Source: three-view drawing plus pictorial views. Frame: mm from the lowest corner of the part. A direction names the side the tool comes from. Coordinates: 2 decimals unless noted, no trailing zeros. Order: outer loops, then holes, each group sorted by start corner. A loop starts at its lowest first (then second) coordinate and runs counter-clockwise, first axis right, second up. Notation, with made-up numbers: (-17, -0.5) -> (25, -0.5) arc R31 ccw to (25, 32.5) -> close; hole circle Ø2 at (36, 63.25). An arc over 180 degrees is marked (long way). One line per question, with ' | ' between items.
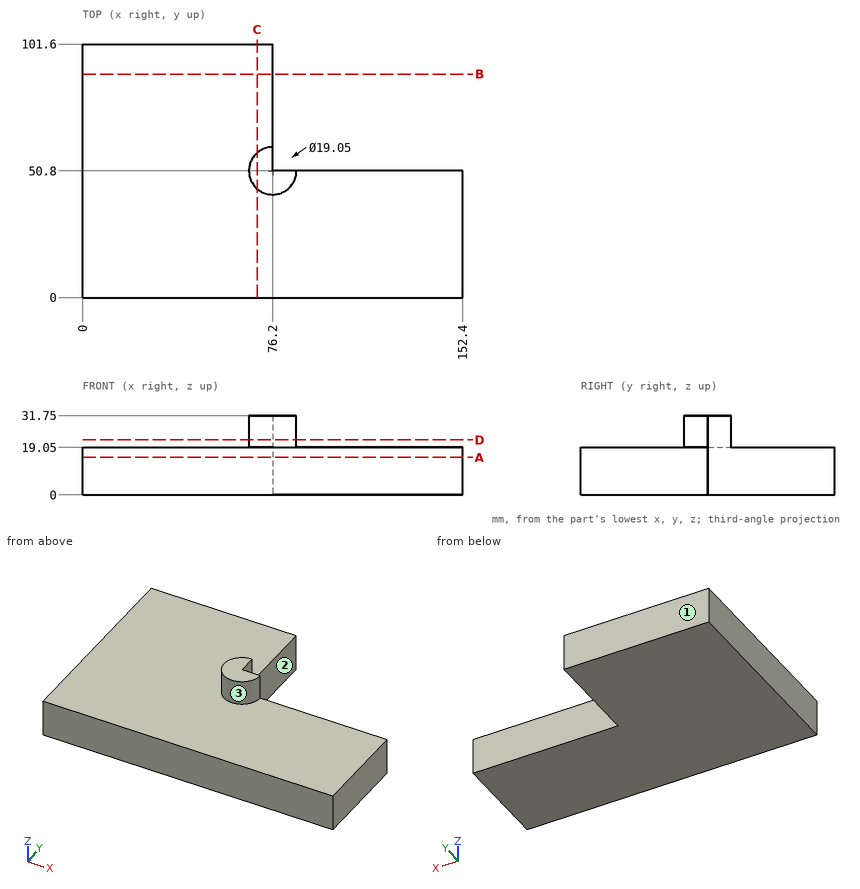
1. Cut plane B-B, the plane y = 89.5. Return loops of the section in (x, z), and give its area (3 significant figures).
Recorded:
outline: (0, 0) -> (76.2, 0) -> (76.2, 19.05) -> (0, 19.05) -> close | area: 1,450 mm^2
2. Access query for the marked faces 1, 2 and 3. Directions: +Z, -Z, +X, -X, +Y, -Y. A direction counts if a zero-diameter tool reaches every point of the face in a straight line with its end or side. Return the directions, or none.
Recorded:
face 1: +Z, -Z, +X, -X, +Y | face 2: +Z, -Z, +X, +Y | face 3: +Z
3. Ray query, line 1 (Z direction, x = 28, y = 63); line 2 (X direction, y = 56.5, z = 9). Return the intervals inside material, ascending. Write a range as [from, to].
Recorded:
line 1: z = [0, 19.05] | line 2: x = [0, 76.2]
4. Cut plane D-D, the plane z = 22. Return loops of the section in (x, y) (3 decimals), and give its area (3 significant figures).
Recorded:
outline: (76.2, 50.8) -> (76.2, 60.325) arc R9.525 ccw (long way) to (85.725, 50.8) -> close | area: 214 mm^2
5. Cut plane C-C, the plane x = 70. Return loops of the section in (y, z).
Recorded:
outline: (0, 0) -> (101.6, 0) -> (101.6, 19.05) -> (58.03, 19.05) -> (58.03, 31.75) -> (43.57, 31.75) -> (43.57, 19.05) -> (0, 19.05) -> close
6. Pin query (flat end, axial travel): pin 1 Ø10 at (x, z) = (123, 19) entering from +Y; pin 2 Ø1 at (x, y) = (26, 49.5) entering from +Z. Return the tip coordinate at first contact, or that it passes through.
Recorded:
pin 1: stops at y = 50.8 | pin 2: stops at z = 19.05
7. Cut plane A-A, the plane z = 15. Return loops of the section in (x, y), and give its area (3 significant figures).
Recorded:
outline: (0, 0) -> (152.4, 0) -> (152.4, 50.8) -> (76.2, 50.8) -> (76.2, 101.6) -> (0, 101.6) -> close | area: 11,600 mm^2
